Verification items for the finished model (mm, model axes). Face numbers are marked on the shaded views. A direction names the side the tool comes from. Round coordinates to 2 decimals unless told otherwise and drop trailing zeros. Write each loop counter-clockwise with the first axis right and the second up, starting at its lowest first coordinate (ties: lowest second). Pieces come first, ordered by that corner, then holes. Notation, with made-up numbers: (84.25, 76.25) - (96.25, 76.25) arc R28 cw to (96.25, 114.25) - close; hole circle Ø4 at (-4, -20). An arc over 180 degrees is marked (long way). Write each question's results on one line, items separated by ' | '.
```python
from build123d import *

# Parameters (mm, degrees)
F2_SIZE  = 0.5
F3_SIZE  = 0.5
F5_DEPTH = 20
F6_W     = 16
F6_H     = 12.5
F7_DEPTH = 15


with BuildPart() as f1:
    # F0 (on Front) → F1 (revolve)
    with BuildSketch(Plane.XZ):
        Polygon((10, 16), (10, 0), (6.1, 0), (6.1, -3), (13, -3), (13, 16), align=None)
    revolve(axis=Axis((0, 0, 6.7583965138), (0, 0, -1)))

    # F2
    f2_edges = [f1.edges().sort_by_distance(p)[0] for p in [
        (-13, 0, 16),
    ]]
    chamfer(f2_edges, length=F2_SIZE)

    # F3
    f3_edges = [f1.edges().sort_by_distance(p)[0] for p in [
        (-10, 0, 16),
    ]]
    chamfer(f3_edges, length=F3_SIZE)

    # F4 (on Front) → F5 (cut)
    with BuildSketch(Plane.XZ):
        Polygon((6.1, 0), (6.1, 5), (0, 5), (-6.1, 5), (-6.1, -5.6750147776), (0, -5.6750147776), (6.1, -5.6750147776), align=None)
    extrude(amount=F5_DEPTH, mode=Mode.SUBTRACT)

    # F6 (on Right) → F7 (cut, symmetric)
    with BuildSketch(Plane.YZ):
        with Locations((-12, 6.25)):
            Rectangle(F6_W, F6_H)
    extrude(amount=F7_DEPTH, both=True, mode=Mode.SUBTRACT)


solid = f1.part
```
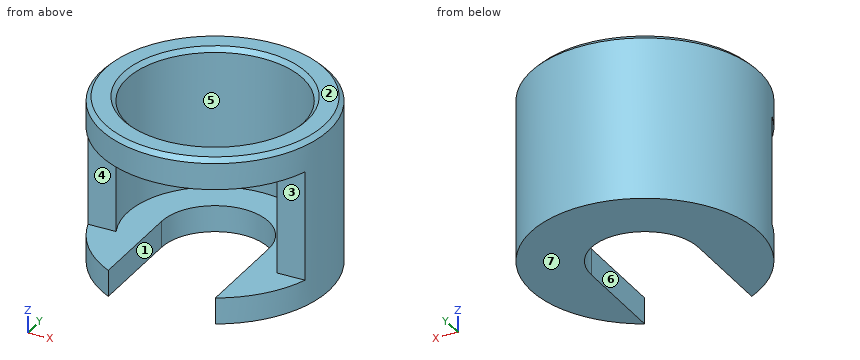
(1) Section check B-B (z = 11). Record the cut outline in (x, y), plus the area to 3 significant figures.
Answer:
outline: (-12.37, -4) - (-9.17, -4) arc R10 cw (long way) to (9.17, -4) - (12.37, -4) arc R13 ccw (long way) to start | area: 133 mm2
(2) Section check A-A (x = 0). Record the cut outline in (y, z).
Answer:
outline: (-13, 12.5) - (-10, 12.5) - (-10, 15.5) - (-10.5, 16) - (-12.5, 16) - (-13, 15.5) - close; (6.1, -3) - (13, -3) - (13, 15.5) - (12.5, 16) - (10.5, 16) - (10, 15.5) - (10, 0) - (6.1, 0) - close
(3) Mould release check, pull along Z, two halves, no side actions. Record for the marked faces 1, 2 and 3: released by +Z, released by -Z, zero draft, split by the parting line, or undercut.
Answer:
face 1: zero draft | face 2: released by +Z | face 3: undercut
(4) Go/stop test with flat-tipped pins: pin 1 Ø8 at (y, z) = (5, 2) entering from +X; pin 2 Ø4.5 at (x, y) = (1, -8.5) entering from -Z; pin 3 Ø0.9 at (y, z) = (-4.5, -1) entering from +X. Record where each tip stops, or that it passes through.
Answer:
pin 1: x = 12.96 | pin 2: z = 12.5 | pin 3: x = 12.35
(5) Thickness scan on L1, parallel to X at y = -0.25, z = 3; L2, parallel to Z at x = -3, y = -11.5; L3, parallel to Y at x = 0, z = 6. Record the ranges inside material, lowest first.
Answer:
L1: -13 to -10, 10 to 13 | L2: 12.5 to 16 | L3: 10 to 13
(6) Set-up check for the marked faces 4, 5, 6 and 7: record each of +Z, -Z, +X, -X, +Y, -Y from which the full face is reachable in a straight line by a thin tool's end or side.
Answer:
face 4: +X, -X, -Y | face 5: +Z | face 6: -Z, -Y | face 7: -Z, +X, -X, +Y, -Y
